Autodesk Inventor part; units mm, degrees
ref_plane "YZ Plane" through (0, 0, 0) normal (1, 0, 0) x (0, 1, 0)
ref_plane "XZ Plane" through (0, 0, 0) normal (0, 1, 0) x (-1, 0, 0)
ref_plane "XY Plane" through (0, 0, 0) normal (0, 0, 1) x (1, 0, 0)
sketch "Skizze1" plane through (0, 0, 0) normal (0, 1, 0) x (-1, 0, 0)
  line L0 (475, 920) -> (-475, 920) construction
  line L1 (-475, 920) -> (-475, -980) construction
  line L2 (475, -980) -> (475, 920) construction
  line L3 (749, 0) -> (-749, 0)
  line L4 (0, -1372) -> (0, 1372)
  line L5 (535, 980) -> (-535, 980)
  line L6 (-535, 980) -> (-535, -980)
  line L7 (535, -980) -> (535, 980)
  line L8 (-535, -980) -> (-475, -980)
  line L9 (475, -980) -> (535, -980)
  line L10 (460, 905) -> (-460, 905)
  line L11 (-460, 905) -> (-460, -980)
  line L12 (460, -980) -> (460, 905)
  line L13 (-475, -980) -> (-460, -980)
  line L14 (460, -980) -> (475, -980)
  dimension "d0" = 1900
  dimension "d1" = 950
  dimension "d2" = 60
  dimension "d3" = 60
  dimension "d4" = 60
  dimension "d7" = 15
  dimension "d8" = 15
  dimension "d9" = 15
extrude "Extrusion1" add sketch "Skizze1" along normal blind 20 contours L7 L9 L14 L12 L3 | L3 L12 L10 L4 L5 L7 | L4 L10 L11 L3 L6 L5 | L11 L13 L8 L6 L3
sketch "Skizze2" plane through (0, 20, 0) normal (0, 1, 0) x (1, 0, 0)
  line L0 (-535, -980) -> (535, -980)
  line L1 (535, -980) -> (535, 980)
  line L2 (535, 980) -> (460, 980)
  line L3 (460, 980) -> (460, -905)
  line L4 (460, -905) -> (-460, -905)
  line L5 (-460, -905) -> (-460, 980)
  line L6 (-460, 980) -> (-535, 980)
  line L7 (-535, 980) -> (-535, -980)
  line L8 (535, 980) -> (460, 980)
  line L9 (475, 980) -> (475, -920)
  line L10 (475, -920) -> (-475, -920)
  line L11 (-475, -920) -> (-475, 980)
  line L12 (0, 1372) -> (0, -1372)
  line L13 (-749, 0) -> (749, 0)
  line L14 (460, 980) -> (460, -905)
  line L15 (475, 980) -> (460, 980)
  line L16 (460, -905) -> (-460, -905)
  line L17 (460, 980) -> (460, -905)
  line L18 (460, -905) -> (-460, -905)
  line L19 (-460, -905) -> (-460, 980)
  line L20 (-460, 980) -> (-535, 980)
  line L21 (-475, 980) -> (-460, 980)
  dimension "d10" = 950
  dimension "d11" = 1900
extrude "Extrusion2" add sketch "Skizze2" along normal blind 100 contours L12 L4 L3 L13 L9 L10 | L10 L11 L13 L5 L4 L12 | L11 L6 L5 L13 | L13 L3 L2 L9
chamfer "Fase1" distance 5 angle 45 6 edges at (-460, 0, -37.5) (0, 0, 905) (460, 0, -37.5) (0, 0, 980) (535, 0, 0) (-535, 0, 0)
mirror "Spiegeln1" about plane through (0, 120, 150.1399) normal (0, 1, 0) of "Extrusion1", "Extrusion2", "Fase1"
equation "\"d3\" = d2"
equation "\"d4\" = d2"
properties part number "Rahmen" material "Holz (Birke)"
Here's how the part is built. I have some questions about the finished solid (model axes, mm). A direction names the side the tool comes from. Give positions to 0.01 mm unless a question says otherwise; leave off trailing zeros. Write each loop counter-clockwise with the first axis right and the second up, starting at its lowest first coordinate (ties: lowest second). Pieces come first, ordered by that corner, then holes.
(1) Thinking about a two-plate mould opening in Y: for faces 1 (the face through (474, 0, 147)), 2 (the face through (-478, 220, 222)), 3 (the face through (460, 118, -24)), which applies, pulls with the +Y half, pulls with the -Y half, needs draft (parallel to the pull), parting line crosses it, or undercut?
Output values:
face 1: pulls with the -Y half
face 2: undercut
face 3: needs draft
(2) If I drill on L1, parallel to X at y = 135, z = 158.5; L2, parallel to Z at x = -381, y = 127.5; L3, parallel to Z at x = -473, y = 36, over which ranges is the centre line in solid material (lowest first)?
Output values:
L1: x = -475 to -460, 460 to 475
L2: z = 905 to 920
L3: z = -980 to 920
(3) Imagine slicing it at B-B, the plane x = -313. Write out the boundary of the cut face in (y, z).
Output values:
outline: (0, 910) - (5, 905) - (235, 905) - (240, 910) - (240, 975) - (235, 980) - (220, 980) - (220, 920) - (20, 920) - (20, 980) - (5, 980) - (0, 975) - close
(4) Will these pins go through, and if not, where does the flat tip stop? pin 1 (2 mm diameter, centred on y = 84, z = 469, fed in from +X); pin 2 (3 mm diameter, centred on y = 209.5, z = 235.5, fed in from -X); pin 3 (12 mm diameter, centred on x = 269.5, y = 74, fed in from +Z).
Output values:
pin 1: stops at x = 475
pin 2: stops at x = -475
pin 3: stops at z = 920
(5) On a 3-axis mill with a long thin cutter (end or side, diameter ignored), from which of +Z, -Z, +X, -X, +Y, -Y can I reach the whole of each face in a straight line? I mean faces 4 (the face through (7, 119, 920)), 5 (the face through (-475, 119, -17)), 6 (the face through (-460, 118, -51)), 7 (the face through (478, 20, 222)), 8 (the face through (475, 119, -43)). Say none if no direction works.
Output values:
face 4: +Z, +X, -X
face 5: +Z, -Z, -X
face 6: -Z, +Y, -Y
face 7: +Z
face 8: +Z, -Z, +X
(6) Imagine slicing it at C-C, the plane y = 93. Write out the boundary of the cut face in (x, z).
Output values:
outline: (-475, -980) - (-460, -980) - (-460, 905) - (460, 905) - (460, -980) - (475, -980) - (475, 920) - (-475, 920) - close
(7) Imagine slicing it at A-A, the plane z = -431. Write out the boundary of the cut face in (x, y).
Output values:
outline: (-535, 5) - (-530, 0) - (-465, 0) - (-460, 5) - (-460, 235) - (-465, 240) - (-530, 240) - (-535, 235) - (-535, 220) - (-475, 220) - (-475, 20) - (-535, 20) - close; (460, 5) - (465, 0) - (530, 0) - (535, 5) - (535, 20) - (475, 20) - (475, 220) - (535, 220) - (535, 235) - (530, 240) - (465, 240) - (460, 235) - close
